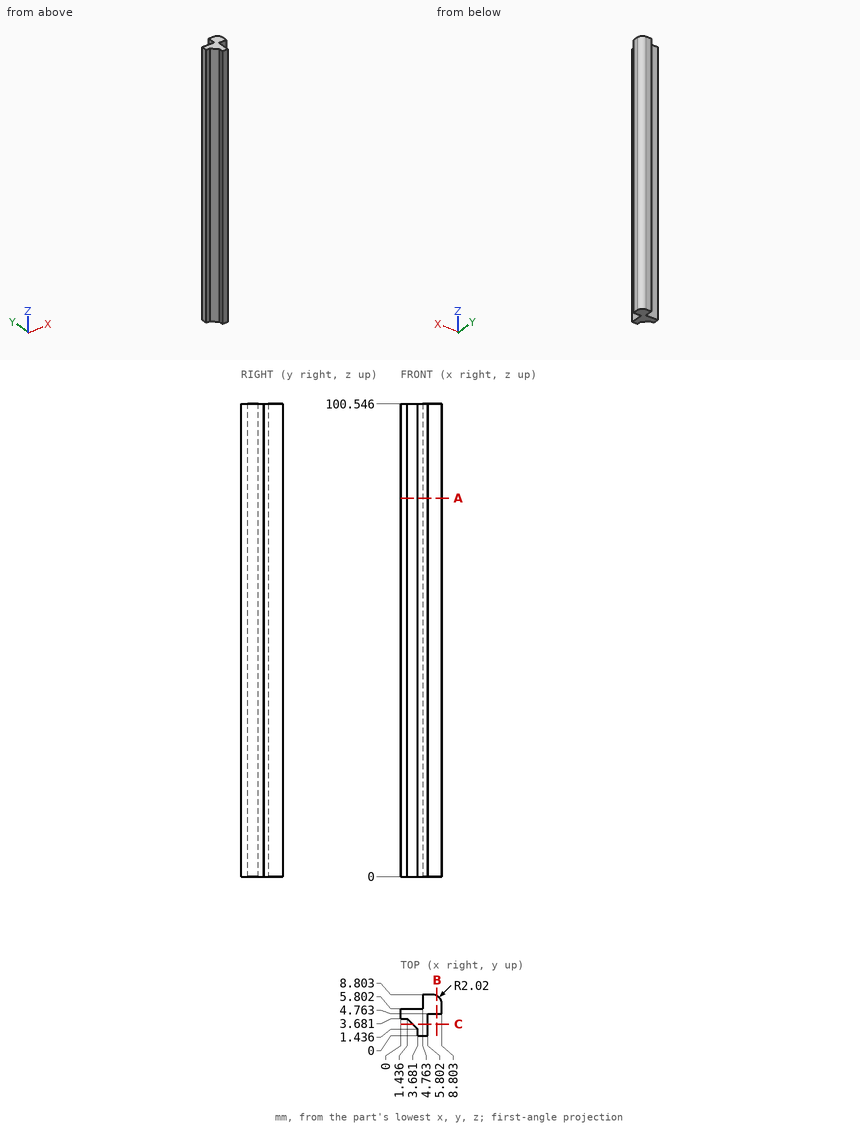
Source: three-view drawing plus pictorial views. Frame: mm from the lowest corner of the part. Give positions to 0.01 mm unless a question says otherwise; leave off trailing zeros. Loops run counter-clockwise (first coordinate to the right, second up) from the corner with the lowest first, then second, coordinate; pieces in that order, holes last. Notation, with made-up numbers: (40, 61) -> (45, 61) arc R21 ccw to (45, 74) -> close; hole circle Ø4 at (-21.5, 22.5). An arc over 180 degrees is marked (long way). Use a Markdown table: item, result. Add a question column.
(1) Ray query, line 1 (Y direction, x = 4, z = 57); line 2 (Y direction, x = 1, z = 17.5). Return the intervals inside material, ascending.
(2) Section query B-B (x = 7.75). Output: boundary loops of the cut face in (y, z) (1 decimal).
(3) Section query C-C (y = 2.5). Output: boundary loops of the cut face in (x, z) (1 decimal).
(4) Section query A-A (z = 80.5). Output: boundary loops of the cut face in (x, y).
(5) First-contact query: pin 1 Ø0.9 at (x, z) = (8, 47) entering from -Y; pin 2 Ø2 at (y, z) = (2.5, 23.5) entering from -X; pin 3 Ø2.5 at (y, z) = (2, 71.5) entering from +X. Flat tips, straight axial feed; report the tip coordinate or a pass-through.
Checked values:
| question | item | result |
|---|---|---|
| 1 | line 1 | 0 to 5.8 |
| 1 | line 2 | 3.68 to 5.8 |
| 2 | outline | (4.8, 0) -> (8.6, 0) -> (8.6, 100.5) -> (4.8, 100.5) -> close |
| 3 | outline | (2.6, 0) -> (5.8, 0) -> (5.8, 100.5) -> (2.6, 100.5) -> close |
| 4 | outline | (0, 3.68) -> (1.44, 3.68) -> (3.68, 1.44) -> (3.68, 0) -> (5.8, 0) -> (5.8, 4.76) -> (8.8, 4.76) -> (8.8, 6.78) arc R2.02 ccw to (6.78, 8.8) -> (4.76, 8.8) -> (4.76, 5.8) -> (0, 5.8) -> close |
| 5 | pin 1 | y = 4.76 |
| 5 | pin 2 | x = 1.62 |
| 5 | pin 3 | x = 5.8 |
